Could you check a few things on this drawing? It's one solid part, dimensions in mm from its lowest x, y, z. A direction names the side the tool comes from. Round coordinates to 2 decimals unless told otherwise and drop trailing zeros. Write each loop counter-clockwise with the first axis right and the second up, starting at its lowest first coordinate (ties: lowest second). Pieces come first, ordered by that corner, then holes. Notation, with made-up numbers: (8.25, -21.75) -> (14.25, -21.75) arc R26 cw to (14.25, 16.25) -> close; hole circle Ø7 at (62, 55). An arc over 180 degrees is marked (long way). Answer as CSV lines item,"result".
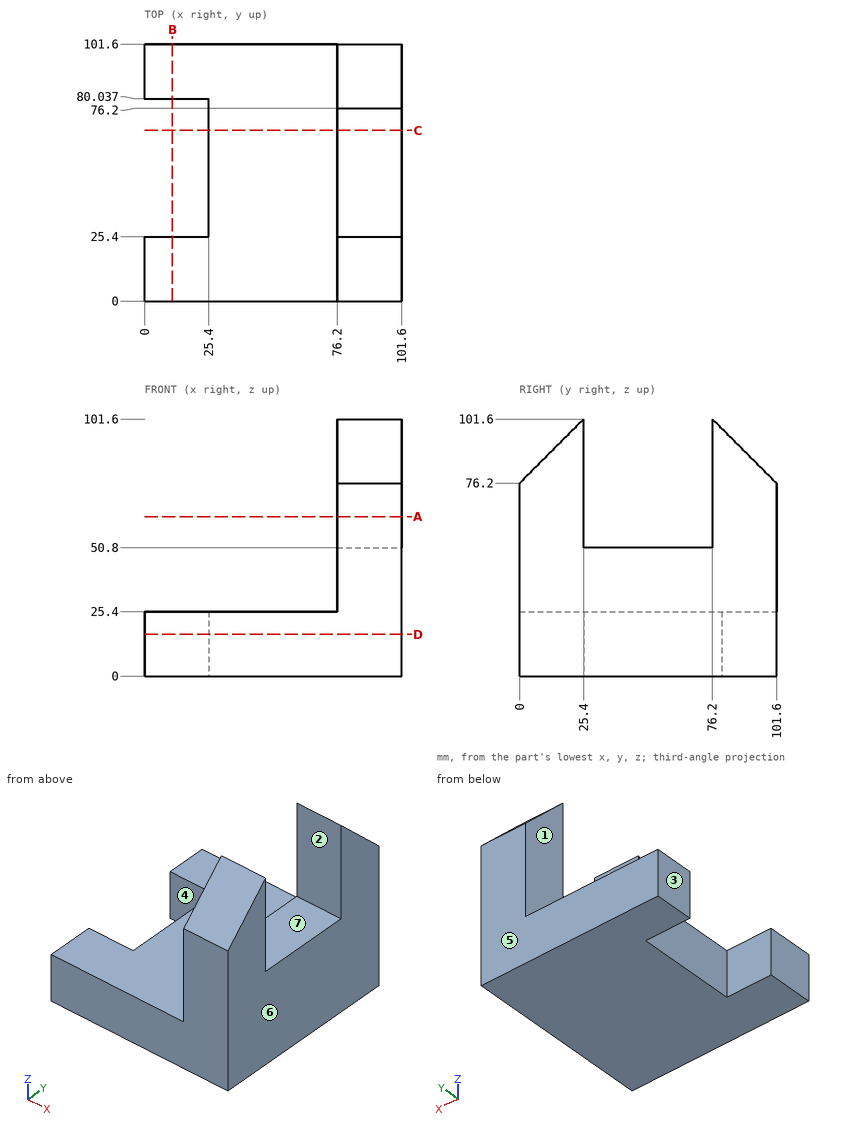
1. Suppose I cut it at A-A on z = 63. Please give me the cut outline in (x, y).
Numbers:
outline,"(76.2, 0) -> (101.6, 0) -> (101.6, 25.4) -> (76.2, 25.4) -> close; (76.2, 76.2) -> (101.6, 76.2) -> (101.6, 101.6) -> (76.2, 101.6) -> close"
2. If we mould it in two halves opening along Y, with no side actions, what happens to the marked faces 5, 6 and 7? For each: released by +Y, released by -Y, zero draft, split by the parting line, or undercut.
Numbers:
face 5,"released by +Y"
face 6,"zero draft"
face 7,"undercut"
3. For pin 1 Ø23 at (y, z) = (66.5, 58.5) entering from -X; pin 2 Ø1 at (x, z) = (75, 31) entering from +Y; pin 3 Ø7.5 at (x, z) = (10, 9) entering from -Y; pin 4 Ø12.5 at (x, y) = (91.5, 60) entering from +Z, each with a flat end and sliding along its axis, tell me the tip position at first contact or that it passes through.
Numbers:
pin 1,"stops at x = 76.2"
pin 2,"passes through"
pin 3,"stops at y = 0"
pin 4,"stops at z = 50.8"
4. Suppose I cut it at C-C on y = 67.5. Please give me the cut outline in (x, z).
Numbers:
outline,"(25.4, 0) -> (101.6, 0) -> (101.6, 50.8) -> (76.2, 50.8) -> (76.2, 25.4) -> (25.4, 25.4) -> close"
5. Suppose I cut it at D-D on z = 16.5. Please give me the cut outline in (x, y).
Numbers:
outline,"(0, 0) -> (101.6, 0) -> (101.6, 101.6) -> (0, 101.6) -> (0, 80.04) -> (25.4, 80.04) -> (25.4, 25.4) -> (0, 25.4) -> close"
6. On a 3-axis mill with a long thin cutter (end or side, diameter ignored), from which of +Z, -Z, +X, -X, +Y, -Y can I reach the whole of each face in a straight line? I mean the marked faces 1, 2, 3 and 4. Say none if no direction works.
Numbers:
face 1,"+Z, -X, +Y, -Y"
face 2,"+Z, +X, -X"
face 3,"+Z, -Z, -X, +Y, -Y"
face 4,"+Z, -Z, -X"
7. If I drill on line 1 (Y direction, x = 78.5, z = 59); line 2 (Y direction, x = 6, z = 23); line 3 (Z direction, x = 65, y = 65.5), over which ranges is the centre line in solid material (lowest first)?
Numbers:
line 1,"y = 0 to 25.4, 76.2 to 101.6"
line 2,"y = 0 to 25.4, 80.04 to 101.6"
line 3,"z = 0 to 25.4"
8. Suppose I cut it at B-B on x = 11. Please give me the cut outline in (y, z).
Numbers:
outline,"(0, 0) -> (25.4, 0) -> (25.4, 25.4) -> (0, 25.4) -> close; (80.04, 0) -> (101.6, 0) -> (101.6, 25.4) -> (80.04, 25.4) -> close"
